Answer from the drawing. Dimensions are ordinates in mm from the lowest x, y and z of the part. Coordinates: 2 decimals unless noted, no trailing zeros. Loops run counter-clockwise (first coordinate to the right, second up) from the corner with the lowest first, then second, coordinate; pieces in that order, holes last. Notation, with made-up numbers: (5.5, -16.75) - (28.5, -16.75) arc R14 cw to (28.5, -9.75) - close; hole circle Ø7 at (-3.5, 27). An arc over 180 degrees is marked (long way). Write each question's results on one line, items separated by ' | '. Start each with the question number.
1. A cutting plane is placed at C-C on x = 2.5. Determine the outline of the cut face in (y, z), then the cut area to 3 significant figures.
2. Find the intervals of material crossed by line 1 along X through (y, z) = (0.75, 0.35) (1 decimal); line 2 along Z through (x, y) = (19.25, 2.35); line 3 along Z through (x, y) = (3, 2.3), in increasing order. Write a range as [from, to].
3. A cutting plane is placed at A-A on y = 4.25. Determine the outline of the cut face in (x, z) (1 decimal).
4. A cutting plane is placed at B-B on z = 1.2. Determine the outline of the cut face in (x, y), then the cut area to 3 significant figures.
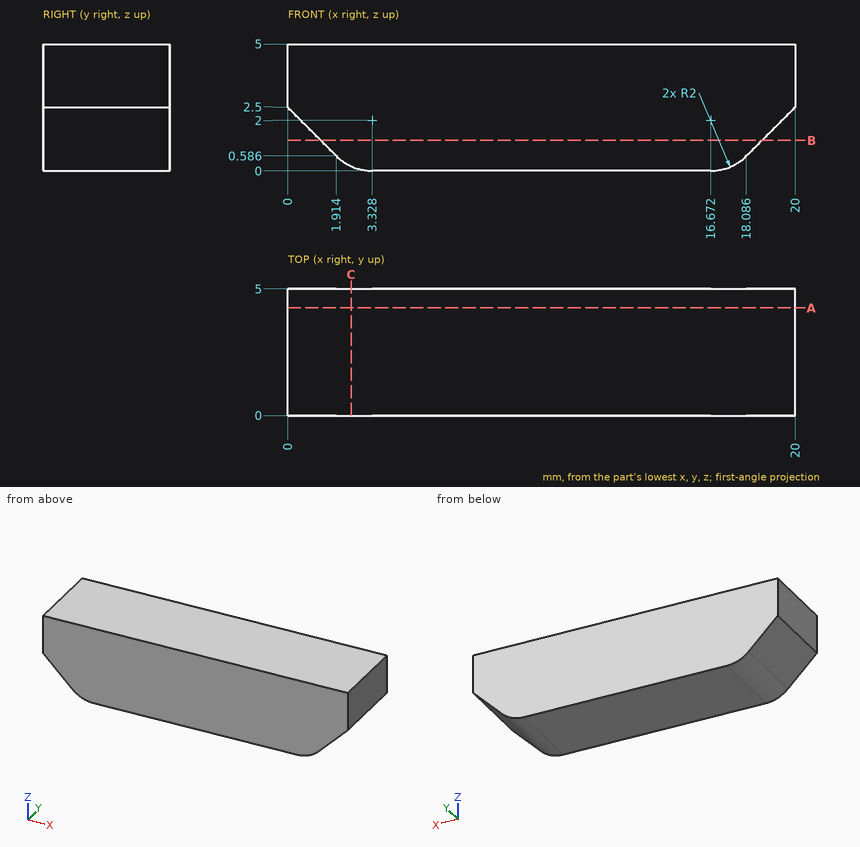
Values:
1) outline: (0, 0.18) - (5, 0.18) - (5, 5) - (0, 5) - close | area: 24.1 mm^2
2) line 1: [2.2, 17.8] | line 2: [1.75, 5] | line 3: [0.03, 5]
3) outline: (0, 2.5) - (1.9, 0.6) arc R2 ccw to (3.3, 0) - (16.7, 0) arc R2 ccw to (18.1, 0.6) - (20, 2.5) - (20, 5) - (0, 5) - close
4) outline: (1.3, 0) - (18.7, 0) - (18.7, 5) - (1.3, 5) - close | area: 87.0 mm^2
